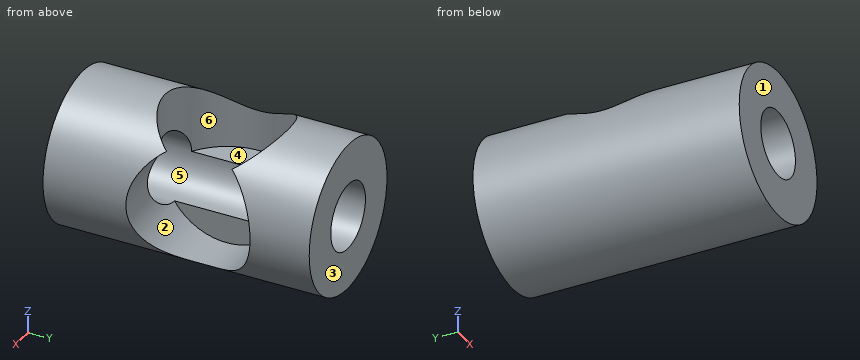
Autodesk Inventor part; units mm, degrees
ref_plane "YZ Plane" through (0, 0, 0) normal (1, 0, 0) x (0, 1, 0)
ref_plane "XZ Plane" through (0, 0, 0) normal (0, 1, 0) x (-1, 0, 0)
ref_plane "XY Plane" through (0, 0, 0) normal (0, 0, 1) x (1, 0, 0)
sketch "Sketch1" plane through (0, 0, 0) normal (0, 1, 0) x (-1, 0, 0)
  circle A0 centre (0, 0) radius 1.125
  circle A1 centre (0, 0) radius 2.525
  dimension "d0" = 2.25
  dimension "d1" = 5.05
extrude "Extrusion1" add sketch "Sketch1" along normal blind 9
sketch "Sketch2" plane through (0, 0, 0) normal (0, 0, 1) x (1, 0, 0)
  line L0 (2.525, 9) -> (-2.525, 9)
  line L1 (2.525, 0) -> (-2.525, 0)
  line L2 (-2.525, 0) -> (-2.525, 9)
  line L3 (-2.525, 7) -> (2.5173, 7)
  line L4 (2.525, 9) -> (-2.525, 9)
  line L5 (0, 9) -> (0, 0)
  circle A0 centre (0, 4.9) radius 2.1
  dimension "d4" = 2
  dimension "d5" = 4.2
extrude "Extrusion2" cut sketch "Sketch2" along normal blind 12 contours A0 L5 | L5 A0
sketch "Sketch3" plane through (0, 0, 0) normal (1, 0, 0) x (0, 1, 0)
  line L0 (9, -2.525) -> (9, 2.525)
  line L1 (0, -2.525) -> (0, 2.525)
  line L2 (0, 2.525) -> (9, 2.525)
  line L3 (7, 2.525) -> (7, -2.525)
  line L4 (9, 1.125) -> (9, -1.125)
  line L5 (9, 0) -> (0, 0)
  circle A0 centre (4.9, 0) radius 2.1
  point P0 (4.9, 1.402)
  dimension "d8" = 2
  dimension "d9" = 4.2
extrude "Extrusion3" cut sketch "Sketch3" along normal up to next contours A0 L5 | L5 A0
properties part number "motor_shaft_adapter" material "ABS Plastic"
Read the model definition and answer for the solid it produces. Units are mm, in the model's axes. Face numbers are marked on the shaded views. A direction names the side the tool comes from. Coordinates: 2 decimals unless noted, no trailing zeros. Write each loop counter-clockwise with the first axis right and the second up, starting at its lowest first coordinate (ties: lowest second). Pieces come first, ordered by that corner, then holes. Notation, with made-up numbers: M 89,47 L 97,47 A13 cw 97,71 Z; hole C 5,-9 d2. An arc over 180 degrees is marked long. Use a Markdown table: item, result.
Q1. Straight lines are drawn through the part: L1, parallel to X at y = 2.5, z = 0 (3 decimals); L2, parallel to Y at x = 1.25, z = 0.05; L3, parallel to Z at x = -0.5, y = 1.25 (3 decimals). For each, find the intervals that lie inside material, in ascending order. Write a range as [from, to].
Answer block:
| item | result |
|---|---|
| L1 | x = [-2.525, -1.125], [1.125, 2.525] |
| L2 | y = [0, 2.8], [7, 9] |
| L3 | z = [-2.475, -1.008], [1.008, 2.475] |
Q2. Each of these flat-tipped pins is pushed along its axis until it touches: pin 1 Ø1.5 at (x, y) = (-1.5, 7) entering from -Z; pin 2 Ø0.5 at (y, z) = (5, -1.5) entering from +X; pin 3 Ø1 at (x, y) = (-1.5, 3.5) entering from -Z. Where does it stop, or does it pass through?
Answer block:
| item | result |
|---|---|
| pin 1 | stops at z = -2.41 |
| pin 2 | stops at x = 0 |
| pin 3 | stops at z = -2.32 |
Q3. The part is cut by section B-B, the plane z = 1.95. Write down the section's boundary in (x, y), then the cut area to 3 significant figures.
Answer block:
| item | result |
|---|---|
| outline | M -1.6,0 L 1.6,0 L 1.6,3.54 A2.1 cw -1.6,3.54 Z; M -1.6,6.26 A2.1 cw 1.6,6.26 L 1.6,9 L -1.6,9 Z |
| area | 16.9 mm2 |
Q4. Which of the six approach directions +Z, -Z, +X, -X, +Y, -Y give full straight-line access (tool end or side, diameter ignored) to the marked faces 4, 5 and 6?
Answer block:
| item | result |
|---|---|
| face 4 | +Z, +X |
| face 5 | +Y, -Y |
| face 6 | +Z |
Q5. Determine the mould class of the marked faces 1, 2 and 3 for opening direction Y: released by +Y, released by -Y, zero draft, split by the parting line, or undercut.
Answer block:
| item | result |
|---|---|
| face 1 | released by -Y |
| face 2 | undercut |
| face 3 | released by +Y |
Q6. The part is cut by section A-A, the plane x = 0.25. Write down the section's boundary in (y, z), then the cut area to 3 significant figures.
Answer block:
| item | result |
|---|---|
| outline | M 0,-2.51 L 9,-2.51 L 9,-1.1 L 6.69,-1.1 A2.1 cw 3.11,-1.1 L 0,-1.1 Z; M 0,1.1 L 2.81,1.1 L 2.81,2.51 L 0,2.51 Z; M 6.99,1.1 L 9,1.1 L 9,2.51 L 6.99,2.51 Z |
| area | 17.0 mm2 |
Q7. The part is cut by section C-C, the plane z = -0.7. Write down the section's boundary in (x, y), then the cut area to 3 significant figures.
Answer block:
| item | result |
|---|---|
| outline | M -2.43,0 L -0.88,0 L -0.88,9 L -2.43,9 Z; M 0.88,0 L 2.43,0 L 2.43,2.92 L 0.88,2.92 Z; M 0.88,6.88 L 2.43,6.88 L 2.43,9 L 0.88,9 Z |
| area | 21.7 mm2 |
Q8. The part is cut by section D-D, the plane y = 2.5. Write down the section's boundary in (x, z) (3 decimals).
Answer block:
| item | result |
|---|---|
| outline | C 0,0 d5.05; hole C 0,0 d2.25 |
